from build123d import *

# Parameters (mm, degrees)
SKETCH_1_R          = 2.25
SKETCH_1_R_2        = 3
EXTRUDE_1_DEPTH     = 1.2
SKETCH_2_R          = 10.7
SKETCH_2_R_2        = 3
EXTRUDE_2_DEPTH     = 6
CUT_EXTRUDE_1_DEPTH = 6


with BuildPart() as part:
    # ｽｹｯﾁ1 → ﾎﾞｽ - 押し出し1 (new body)
    with BuildSketch(Plane.XY):
        with BuildLine():
            Line((-10.949386038, 8.724158721), (0, 22.466349623))
            Line((0, 22.466349623), (10.148136548, 9.644445272))
            ThreePointArc((10.148136548, 9.644445272), (14, 0), (10.148136548, -9.644445272))
            Line((10.148136548, -9.644445272), (0, -22.466349623))
            Line((0, -22.466349623), (-10.949386038, -8.724158721))
            ThreePointArc((-10.949386038, -8.724158721), (-14, 0), (-10.949386038, 8.724158721))
        make_face()
        with Locations((0, 15)):
            Circle(SKETCH_1_R, mode=Mode.SUBTRACT)
        with Locations((0, -15)):
            Circle(SKETCH_1_R, mode=Mode.SUBTRACT)
        Circle(SKETCH_1_R_2, mode=Mode.SUBTRACT)
    extrude(amount=EXTRUDE_1_DEPTH)

    # ｽｹｯﾁ2 → ﾎﾞｽ - 押し出し2 (add)
    with BuildSketch(Plane.XY.offset(1.2)):
        Circle(SKETCH_2_R)
        Circle(SKETCH_2_R_2, mode=Mode.SUBTRACT)
    extrude(amount=EXTRUDE_2_DEPTH)

    # ｽｹｯﾁ3 → ｶｯﾄ - 押し出し1 (cut)
    with BuildSketch(Plane.XY.offset(1.2)):
        Polygon((-2.565036178, 19.24706256), (2.547965093, 19.24706256), (0, 22.466349623), align=None)
        Polygon((-2.565036178, -19.24706256), (2.547965093, -19.24706256), (0, -22.466349623), align=None)
    extrude(amount=-CUT_EXTRUDE_1_DEPTH, mode=Mode.SUBTRACT)


solid = part.part
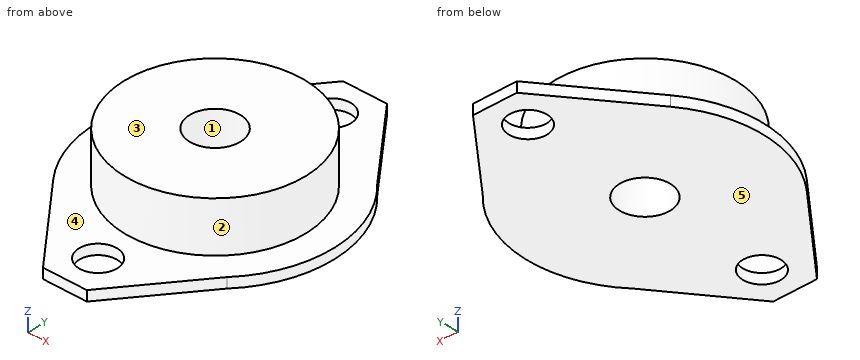
For this review, take the finished solid that the model builds, in its own axes (mm). Face numbers are marked on the shaded views. A direction names the side the tool comes from. Round coordinates to 2 decimals unless told otherwise and drop trailing zeros. Write each loop counter-clockwise with the first axis right and the second up, starting at its lowest first coordinate (ties: lowest second). Pieces come first, ordered by that corner, then holes. Notation, with made-up numbers: (45.25, 18.25) -> (62.25, 18.25) arc R28 cw to (62.25, 39.25) -> close; hole circle Ø10 at (52, 39.25). An arc over 180 degrees is marked (long way). Use CSV: the item, a comma, the result in double quotes.
(1) Draft analysis for pull direction X (two halves, no side actions). For the marked faces 1, 2 and 3, state which applies: +X half, -X half, draft (parallel to the pull), parting line (faces both ways), or undercut.
Computed values:
face 1,"undercut"
face 2,"parting line"
face 3,"draft"
(2) Consider section D-D, the plane y = -15.5. Give the boundary of the cut face in (x, z), plus the area to 3 significant figures.
Computed values:
outline,"(-5.55, 0) -> (-2.19, 0) -> (-2.19, 1.2) -> (-5.55, 1.2) -> close; (2.19, 0) -> (5.51, 0) -> (5.51, 1.2) -> (2.19, 1.2) -> close"
area,"8.01 mm²"
(3) Consider section A-A, the plane x = 0. Give the boundary of the cut face in (y, z).
Computed values:
outline,"(-19.25, 0) -> (-17.25, 0) -> (-17.25, 1.2) -> (-19.25, 1.2) -> close; (-12.75, 0) -> (-3, 0) -> (-3, 7.2) -> (-10.7, 7.2) -> (-10.7, 1.2) -> (-12.75, 1.2) -> close; (3, 0) -> (12.75, 0) -> (12.75, 1.2) -> (10.7, 1.2) -> (10.7, 7.2) -> (3, 7.2) -> close; (17.25, 0) -> (19.25, 0) -> (19.25, 1.2) -> (17.25, 1.2) -> close"
(4) Clearance check with flat-ended pins moving along their axes: P1, Ø1.5, axis at x = 5, z = 4.5, coming from the -Y side; P2, Ø1.5, axis at x = 3, y = 4, coming from the -Z side; P3, Ø5, axis at x = -2.5, y = 13, coming from the +Z side. State where each tip first meets the part, or that it passes through.
Computed values:
P1,"y = -9.82"
P2,"z = 0"
P3,"z = 1.2"
(5) Consider section B-B, the plane y = 0. Give the boundary of the cut face in (x, z), plus the area to 3 significant figures.
Computed values:
outline,"(-14, 0) -> (-3, 0) -> (-3, 7.2) -> (-10.7, 7.2) -> (-10.7, 1.2) -> (-14, 1.2) -> close; (3, 0) -> (14, 0) -> (14, 1.2) -> (10.7, 1.2) -> (10.7, 7.2) -> (3, 7.2) -> close"
area,"119 mm²"
(6) Consider section C-C, the plane z = 0.5. Give the boundary of the cut face in (x, y).
Computed values:
outline,"(-10.95, -8.72) -> (-2.57, -19.25) -> (2.55, -19.25) -> (10.15, -9.64) arc R14 ccw to (10.15, 9.64) -> (2.55, 19.25) -> (-2.57, 19.25) -> (-10.95, 8.72) arc R14 ccw to start; hole circle Ø6 at (0, 0); hole circle Ø4.5 at (0, -15); hole circle Ø4.5 at (0, 15)"
(7) For the marked faces 4 and 5, list the 3-axis set-ups (+Z, -Z, +X, -X, +Y, -Y) from which the entire face can be reached by the end or side of a thin tool; tool diameter is ignored.
Computed values:
face 4,"+Z"
face 5,"-Z, +X, -X, +Y, -Y"
(8) To check wall thickness, follow L1, parallel to Y at x = 0, z = 0.4; L2, parallel to Y at x = 0, z = 3.5; L3, parallel to Z at x = 8, y = -10. State the ranges of each line that lie inside material, in increasing order. Write a range as [from, to].
Computed values:
L1,"[-19.25, -17.25], [-12.75, -3], [3, 12.75], [17.25, 19.25]"
L2,"[-10.7, -3], [3, 10.7]"
L3,"[0, 1.2]"
